Design review of the part built by this model. Coordinates are the model's own, in mm. Coordinates: 2 decimals unless noted, no trailing zeros. Order: outer loops, then holes, each group sorted by start corner. A loop starts at its lowest first (then second) coordinate and runs counter-clockwise, first axis right, second up. Notation, with made-up numbers: M -18,-32 L 34,-32 A25 ccw 34,-2 Z; hole C -26.75,27.25 d10. An arc over 180 degrees is marked long. Answer as a JSON object with one key per item and string values.
from build123d import *

# Parameters (mm, degrees)
SKETCH_1_W          = 150
SKETCH_1_H          = 230
EXTRUDE_1_DEPTH     = 3
SKETCH_2_R          = 1.6
CUT_EXTRUDE_1_DEPTH = 275.606991899
SKETCH_3_R          = 1.6
CUT_EXTRUDE_2_DEPTH = 275.606991899
CUT_EXTRUDE_3_REACH = 276.607
CUT_EXTRUDE_4_REACH = 276.607
SKETCH_5_W          = 49.5
SKETCH_5_H          = 163.5
FILLET_1_R          = 4
CUT_EXTRUDE_6_REACH = 276.607
SKETCH_7_R          = 1.25
FILLET_3_R          = 1
CUT_EXTRUDE_7_REACH = 276.607
SKETCH_8_W          = 20
SKETCH_8_H          = 31
FILLET_4_R          = 3
SKETCH_9_R          = 2.75
CUT_EXTRUDE_8_DEPTH = 275.606991899


with BuildPart() as part:
    # 草图1 → 凸台-拉伸1 (new body)
    with BuildSketch(Plane.XY):
        with Locations((75, 115)):
            Rectangle(SKETCH_1_W, SKETCH_1_H)
    extrude(amount=EXTRUDE_1_DEPTH)

    # 草图2 → 切除-拉伸1 (cut, through all)
    with BuildSketch(Plane.XY.offset(3)):
        with Locations((86.5, 20)):
            Circle(SKETCH_2_R)
        with Locations((86.5, 40)):
            Circle(SKETCH_2_R)
        with Locations((86.5, 155)):
            Circle(SKETCH_2_R)
        with Locations((86.5, 175)):
            Circle(SKETCH_2_R)
        with Locations((5, 10)):
            Circle(SKETCH_2_R)
        with Locations((143, 8)):
            Circle(SKETCH_2_R)
        with Locations((143, 188)):
            Circle(SKETCH_2_R)
        with Locations((5, 170)):
            Circle(SKETCH_2_R)
        with Locations((5, 190)):
            Circle(SKETCH_2_R)
        with Locations((65, 225)):
            Circle(SKETCH_2_R)
        with Locations((85, 225)):
            Circle(SKETCH_2_R)
        with Locations((145, 150)):
            Circle(SKETCH_2_R)
        with Locations((145, 130)):
            Circle(SKETCH_2_R)
    extrude(amount=-CUT_EXTRUDE_1_DEPTH, mode=Mode.SUBTRACT)

    # 草图3 → 切除-拉伸2 (cut, through all)
    with BuildSketch(Plane.XY.offset(3)):
        with Locations((40.19, 34.5)):
            Circle(SKETCH_3_R)
        with Locations(Location((60.19, 34.5, 0), (0, 0, 180))):
            Circle(SKETCH_3_R)
        with BuildLine():
            Line((28, 42), (69, 42))
            ThreePointArc((69, 42), (70.25, 40.75), (69, 39.5))
            Line((69, 39.5), (28, 39.5))
            ThreePointArc((28, 39.5), (26.75, 40.75), (28, 42))
        make_face()
    extrude(amount=-CUT_EXTRUDE_2_DEPTH, mode=Mode.SUBTRACT)

    # 草图4 → 切除-拉伸3 (cut, up to next)
    with BuildSketch(Plane.XY.offset(3), mode=Mode.PRIVATE) as cut_extrude_3_sk1:
        with BuildLine():
            Line((56.69, 135), (64.69, 135))
            ThreePointArc((64.69, 135), (66.104213562, 134.414213562), (66.69, 133))
            Line((66.69, 133), (66.69, 47))
            ThreePointArc((66.69, 47), (66.104213562, 45.585786438), (64.69, 45))
            Line((64.69, 45), (56.69, 45))
            ThreePointArc((56.69, 45), (55.275786438, 45.585786438), (54.69, 47))
            Line((54.69, 47), (54.69, 133))
            ThreePointArc((54.69, 133), (55.275786438, 134.414213562), (56.69, 135))
        make_face()
    cut_extrude_3_tool1 = extrude(cut_extrude_3_sk1.sketch, amount=-CUT_EXTRUDE_3_REACH, mode=Mode.PRIVATE) & part.part
    add(cut_extrude_3_tool1.solids().sort_by_distance((60.69, 90, 3))[0], mode=Mode.SUBTRACT)

    # 草图5 → 切除-拉伸4 (cut, up to next)
    with BuildSketch(Plane.XY.offset(3), mode=Mode.PRIVATE) as cut_extrude_4_sk1:
        with Locations((113.25, 101.75)):
            Rectangle(SKETCH_5_W, SKETCH_5_H)
    cut_extrude_4_tool1 = extrude(cut_extrude_4_sk1.sketch, amount=-CUT_EXTRUDE_4_REACH, mode=Mode.PRIVATE) & part.part
    add(cut_extrude_4_tool1.solids().sort_by_distance((113.25, 101.75, 3))[0], mode=Mode.SUBTRACT)

    # 圆角1
    fillet_1_edges = [part.edges().sort_by_distance(p)[0] for p in [
        (0, 230, 1.5),
        (150, 230, 1.5),
    ]]
    fillet(fillet_1_edges, radius=FILLET_1_R)

    # 草图7 → 切除-拉伸6 (cut, up to next)
    with BuildSketch(Plane.XY.offset(3), mode=Mode.PRIVATE) as cut_extrude_6_sk1:
        with Locations((68, 204)):
            Circle(SKETCH_7_R)
    cut_extrude_6_tool1 = extrude(cut_extrude_6_sk1.sketch, amount=-CUT_EXTRUDE_6_REACH, mode=Mode.PRIVATE) & part.part
    # 草图7 → 切除-拉伸6 (cut, up to next)
    with BuildSketch(Plane.XY.offset(3), mode=Mode.PRIVATE) as cut_extrude_6_sk2:
        with Locations((68, 164)):
            Circle(SKETCH_7_R)
    cut_extrude_6_tool2 = extrude(cut_extrude_6_sk2.sketch, amount=-CUT_EXTRUDE_6_REACH, mode=Mode.PRIVATE) & part.part
    # 草图7 → 切除-拉伸6 (cut, up to next)
    with BuildSketch(Plane.XY.offset(3), mode=Mode.PRIVATE) as cut_extrude_6_sk3:
        Polygon((77.775, 170.1), (77.775, 197.9), (64.620745433, 197.9), (58.225, 191.956783725), (58.225, 176.043216275), (64.620745433, 170.1), align=None)
    cut_extrude_6_tool3 = extrude(cut_extrude_6_sk3.sketch, amount=-CUT_EXTRUDE_6_REACH, mode=Mode.PRIVATE) & part.part
    add(cut_extrude_6_tool1.solids().sort_by_distance((68, 204, 3))[0], mode=Mode.SUBTRACT)
    add(cut_extrude_6_tool2.solids().sort_by_distance((68, 164, 3))[0], mode=Mode.SUBTRACT)
    add(cut_extrude_6_tool3.solids().sort_by_distance((68.574749, 184, 3))[0], mode=Mode.SUBTRACT)

    # 圆角3
    fillet_3_edges = [part.edges().sort_by_distance(p)[0] for p in [
        (138, 183.5, 1.5),
        (138, 20, 1.5),
        (88.5, 20, 1.5),
        (88.5, 183.5, 1.5),
    ]]
    fillet(fillet_3_edges, radius=FILLET_3_R)

    # 草图8 → 切除-拉伸7 (cut, up to next)
    with BuildSketch(Plane.XY.offset(3), mode=Mode.PRIVATE) as cut_extrude_7_sk1:
        with Locations((68, 184)):
            Rectangle(SKETCH_8_W, SKETCH_8_H)
    cut_extrude_7_tool1 = extrude(cut_extrude_7_sk1.sketch, amount=-CUT_EXTRUDE_7_REACH, mode=Mode.PRIVATE) & part.part
    add(cut_extrude_7_tool1.solids().sort_by_distance((68, 184, 3))[0], mode=Mode.SUBTRACT)

    # 圆角4
    fillet_4_edges = [part.edges().sort_by_distance(p)[0] for p in [
        (78, 199.5, 1.5),
        (78, 168.5, 1.5),
        (58, 168.5, 1.5),
        (58, 199.5, 1.5),
    ]]
    fillet(fillet_4_edges, radius=FILLET_4_R)

    # 草图9 → 切除-拉伸8 (cut, through all)
    with BuildSketch(Plane.XY.offset(3)):
        with Locations((74, 150)):
            Circle(SKETCH_9_R)
        with Locations((74, 22)):
            Circle(SKETCH_9_R)
    extrude(amount=-CUT_EXTRUDE_8_DEPTH, mode=Mode.SUBTRACT)


solid = part.part
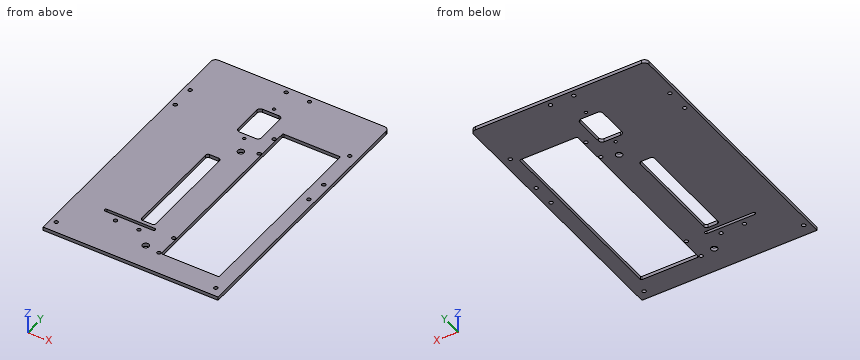
1) Add section A-A (y = 99). State the section outline as (x, z) points, and give its area (4 significant figures).
Taken from the geometry:
{"outline": "M 0,0 L 54.69,0 L 54.69,3 L 0,3 Z; M 66.69,0 L 88.5,0 L 88.5,3 L 66.69,3 Z; M 138,0 L 150,0 L 150,3 L 138,3 Z", "area": "265.5 mm2"}
2) Insertion check: pin 1 Ø1.5 at (x, y) = (68, 164) entering from -Z (3 decimals). The pin has a flat end and moves straight along its axis. Give the tip position at first contact, or say it passes through.
Taken from the geometry:
{"pin 1": "passes through"}
3) Add section C-C (z = 0.7). Count the separate pieces of the cut face and the enclosed holes in it, and give its area (3 significant figures).
Taken from the geometry:
{"separate pieces": "1", "enclosed holes": "23", "area": "24,400 mm2"}
4) To check wall thickness, follow L1, parallel to X at y = 172, z = 2.4; L2, parallel to X at y = 225, z = 2.1; L3, parallel to Y at x = 5, z = 1.2. State the ranges of each line that lie inside material, in increasing order.
Taken from the geometry:
{"L1": "x = 0 to 58, 78 to 88.5, 138 to 150", "L2": "x = 0 to 63.4, 66.6 to 83.4, 86.6 to 150", "L3": "y = 0 to 8.4, 11.6 to 168.4, 171.6 to 188.4, 191.6 to 230"}
5) Add section B-B (x = 134.5). State the section outline as (y, z) points.
Taken from the geometry:
{"outline": "M 0,0 L 20,0 L 20,3 L 0,3 Z; M 183.5,0 L 230,0 L 230,3 L 183.5,3 Z"}
